The listing builds one solid part. Answer for the finished solid, in the listing's coordinates (mm). A direction names the side the tool comes from. Give positions to 0.01 mm unless a question says otherwise; leave off trailing zeros. Write each loop counter-clockwise with the first axis right and the second up, starting at its lowest first coordinate (ties: lowest second). Pieces come first, ordered by that corner, then holes.
```python
from build123d import *

# Parameters (mm, degrees)
F0_W     = 15
F0_H     = 20
F1_DEPTH = 4
F2_R     = 2
F3_DEPTH = 19
F4_R     = 3.25
F4_R_2   = 2
F5_DEPTH = 5
F6_W     = 7
F6_H     = 4
F7_DEPTH = 15.001
F8_W     = 5
F8_H     = 20
F9_DEPTH = 8.001


with BuildPart() as f1:
    # F0 (on Front) → F1 (new body, symmetric)
    with BuildSketch(Plane.XZ):
        Rectangle(F0_W, F0_H)
    extrude(amount=F1_DEPTH, both=True)

    # F2 (on face) → F3 (cut)
    with BuildSketch(Plane.XY.offset(10)):
        with Locations((-2.5, 0)):
            Circle(F2_R)
    extrude(amount=-F3_DEPTH, mode=Mode.SUBTRACT)

    # F4 (on face) → F5 (cut)
    with BuildSketch(Plane.XY.offset(10)):
        with Locations((-2.5, 0)):
            Circle(F4_R)
        with Locations((-2.5, 0)):
            Circle(F4_R_2, mode=Mode.SUBTRACT)
    extrude(amount=-F5_DEPTH, mode=Mode.SUBTRACT)

    # F6 (on face) → F7 (cut, through all)
    with BuildSketch(Plane.YZ.offset(7.5)):
        with Locations((0, 2.5)):
            Rectangle(F6_W, F6_H)
        with Locations((0, -6.5)):
            Rectangle(F6_W, F6_H)
    extrude(amount=-F7_DEPTH, mode=Mode.SUBTRACT)

    # F8 (on face) → F9 (cut, through all)
    with BuildSketch(Plane.XZ.offset(4)):
        with Locations((5, 0)):
            Rectangle(F8_W, F8_H)
    extrude(amount=-F9_DEPTH, mode=Mode.SUBTRACT)


solid = f1.part
```
Item 1: Consider probe 1 along Z at (x, y) = (-5, -1); probe 2 along Z at (x, y) = (1.75, 2.75); probe 3 along Y at (x, z) = (-6.5, -5.5). Determine where each line is inside the solid, lowest interval first.
Conclusion:
probe 1: z = -10 to -8.5, -4.5 to 0.5, 4.5 to 5
probe 2: z = -10 to -8.5, -4.5 to 0.5, 4.5 to 10
probe 3: y = -4 to -3.5, 3.5 to 4
Item 2: A cutting plane is placed at C-C, the plane z = -2.25. Give the vertices of the cut face in (x, y).
Conclusion:
outline: (-7.5, -4) - (2.5, -4) - (2.5, 4) - (-7.5, 4) - close; hole circle Ø4 at (-2.5, 0)
Item 3: Which of the six approach directions +Z, -Z, +X, -X, +Y, -Y give full straight-line access (tool end or side, diameter ignored) to faces 4 (the face through (-6, 0, 10)), 5 (the face through (-3, 0, -9)), 6 (the face through (-2, 3.5, -7))?
Conclusion:
face 4: +Z, +X, -X, +Y, -Y
face 5: +Z
face 6: +X, -X
Item 4: Each of these flat-tipped pins is pushed along its axis until it touches: P1, Ø4, axis at x = -0.5, y = 1, coming from the +Z side; P2, Ø4.5, axis at x = -2, y = 0, coming from the +Z side. Where does it stop, or does it pass through?
Conclusion:
P1: stops at z = 10
P2: stops at z = 5
Item 5: Determine the mould class of faces 1 (the face through (2.5, 0, 0)), 2 (the face through (0, 0, -8.5)), 3 (the face through (0.6, 0.98, 7.54)) for opening direction X: pulls with the +X half, pulls with the -X half, needs draft (parallel to the pull), parting line crosses it, or undercut.
Conclusion:
face 1: pulls with the +X half
face 2: needs draft
face 3: undercut
Item 6: A cutting plane is placed at A-A, the plane y = 0. Give the vertices of the cut face in (x, z).
Conclusion:
outline: (-7.5, -10) - (2.5, -10) - (2.5, -8.5) - (-0.5, -8.5) - (-0.5, -9) - (-4.5, -9) - (-4.5, -8.5) - (-7.5, -8.5) - close; (-7.5, -4.5) - (-4.5, -4.5) - (-4.5, 0.5) - (-7.5, 0.5) - close; (-7.5, 4.5) - (-4.5, 4.5) - (-4.5, 5) - (-5.75, 5) - (-5.75, 10) - (-7.5, 10) - close; (-0.5, -4.5) - (2.5, -4.5) - (2.5, 0.5) - (-0.5, 0.5) - close; (-0.5, 4.5) - (2.5, 4.5) - (2.5, 10) - (0.75, 10) - (0.75, 5) - (-0.5, 5) - close
Item 7: A cutting plane is placed at B-B, the plane x = 0.5. Give the vertices of the cut face in (y, z), plus the area to 3 significant figures.
Conclusion:
outline: (-4, -10) - (4, -10) - (4, 10) - (1.25, 10) - (1.25, 5) - (-1.25, 5) - (-1.25, 10) - (-4, 10) - close; hole (-3.5, -8.5) - (3.5, -8.5) - (3.5, -4.5) - (-3.5, -4.5) - close; hole (-3.5, 0.5) - (3.5, 0.5) - (3.5, 4.5) - (-3.5, 4.5) - close
area: 91.5 mm2
Item 8: A cutting plane is placed at D-D, the plane x = -2.5. Give the vertices of the cut face in (y, z).
Conclusion:
outline: (-4, -10) - (4, -10) - (4, 10) - (3.25, 10) - (3.25, 5) - (2, 5) - (2, 4.5) - (3.5, 4.5) - (3.5, 0.5) - (2, 0.5) - (2, -4.5) - (3.5, -4.5) - (3.5, -8.5) - (2, -8.5) - (2, -9) - (-2, -9) - (-2, -8.5) - (-3.5, -8.5) - (-3.5, -4.5) - (-2, -4.5) - (-2, 0.5) - (-3.5, 0.5) - (-3.5, 4.5) - (-2, 4.5) - (-2, 5) - (-3.25, 5) - (-3.25, 10) - (-4, 10) - close
